```python
from build123d import *

# Parameters (mm, degrees)
PAD_DEPTH         = 6
PAD001_DEPTH      = 2
PAD002_DEPTH      = 100
SKETCH003_W       = 2.4
SKETCH003_H       = 10
POCKET_DEPTH      = 2.351
POCKET_DEPTH_BACK = -2.351
PAD003_DEPTH      = 10


with BuildPart() as part:
    # Sketch → Pad (new body)
    with BuildSketch(Plane.XY):
        with BuildLine():
            ThreePointArc((-2.3, 2.35), (-3.288237, 0), (-2.3, -2.35))
            Line((-2.3, -2.35), (2.3, -2.35))
            ThreePointArc((2.3, -2.35), (3.288237, 0), (2.3, 2.35))
            Line((-2.3, 2.35), (2.3, 2.35))
        make_face()
        with BuildLine():
            ThreePointArc((1.341641, -1.55), (2.05, 0), (1.341641, 1.55))
            Line((-1.341641, 1.55), (1.341641, 1.55))
            ThreePointArc((-1.341641, 1.55), (-2.05, 0), (-1.341641, -1.55))
            Line((1.341641, -1.55), (-1.341641, -1.55))
        make_face(mode=Mode.SUBTRACT)
    extrude(amount=PAD_DEPTH)

    # Sketch001 → Pad001 (join)
    with BuildSketch(Plane.XY):
        with BuildLine():
            ThreePointArc((-2.3, 2.3), (-3.252691, 0), (-2.3, -2.3))
            Line((-2.3, -2.3), (2.3, -2.3))
            ThreePointArc((2.3, -2.3), (3.252691, 0), (2.3, 2.3))
            Line((-2.3, 2.3), (2.3, 2.3))
        make_face()
    extrude(amount=-PAD001_DEPTH)

    # Sketch002 → Pad002 (join)
    with BuildSketch(Plane.XY.offset(-2)):
        Polygon((-0.8, 2.35), (-0.8, -0.75), (-2.3, -0.75), (-2.3, -2.35), (2.3, -2.35), (2.3, -0.75), (0.8, -0.75), (0.8, 2.35), align=None)
    extrude(amount=-PAD002_DEPTH)

    # Sketch003 → Pocket (cut, two sides)
    with BuildSketch(Plane.XZ) as pocket_sk:
        with Locations((0, 5)):
            Rectangle(SKETCH003_W, SKETCH003_H)
    extrude(amount=-POCKET_DEPTH, mode=Mode.SUBTRACT)
    extrude(pocket_sk.sketch, amount=-POCKET_DEPTH_BACK, mode=Mode.SUBTRACT)

    # Sketch004 → Pad003 (join)
    with BuildSketch(Plane.XY.offset(-102)):
        with BuildLine():
            ThreePointArc((2.12132, 4.12132), (2.771639, 5.09459), (3, 6.242641))
            Line((3, 16.242641), (3, 6.242641))
            ThreePointArc((3, 16.242641), (2.771639, 17.390691), (2.12132, 18.363961))
            Line((2.12132, 18.363961), (1.375736, 19.109545))
            ThreePointArc((2.224264, 19.958074), (1.375736, 19.958074), (1.375736, 19.109545))
            Line((2.969848, 19.212489), (2.224264, 19.958074))
            ThreePointArc((4.2, 16.242641), (3.880294, 17.849911), (2.969848, 19.212489))
            Line((4.2, 16.242641), (4.2, 6.242641))
            ThreePointArc((2.969848, 3.272792), (3.880294, 4.63537), (4.2, 6.242641))
            Line((2.969848, 3.272792), (0, 0.302944))
            Line((0, 2), (0, 0.302944))
            Line((2.12132, 4.12132), (0, 2))
        make_face()
    pad003 = extrude(amount=PAD003_DEPTH)

    # Mirrored: Pad003 across Sketch004 V_Axis
    add(pad003.mirror(Plane(origin=(0, 0, -102), x_dir=(0, 0, 1), z_dir=(1, 0, 0))))


solid = part.part
```
Input: part model. Units: mm. Frame: model coordinates. A direction names the side the tool comes from. Give positions to 0.01 mm unless a question says otherwise; leave off trailing zeros. Order: outer loops, then holes, each group sorted by start corner. A loop starts at its lowest first (then second) coordinate and runs counter-clockwise, first axis right, second up. Notation, with made-up numbers: M -25,-5 L 15,-5 A18 ccw 15,0 Z; hole C 8,8 d8. An arc over 180 degrees is marked long. Return JSON: item names as keys, results as strings.
1) Contact query for flat-ended pins moving along their axis: pin 1 (6 mm diameter, centred on y = 6.5, z = -21, fed in from +X); pin 2 (4.5 mm diameter, centred on x = 0, y = -0.5, fed in from +Z); pin 3 (0.5 mm diameter, centred on y = -1.5, z = -65, fed in from +X); pin 4 (0.9 mm diameter, centred on y = 2, z = 2, fed in from +X). Output: stop coordinate, or through.
Taken from the geometry:
{"pin 1": "passes through", "pin 2": "stops at z = 6", "pin 3": "stops at x = 2.3", "pin 4": "stops at x = 2.9"}
2) Section query C-C on y = 17.25. Output: boundary loops of the cut face in (x, z).
Taken from the geometry:
{"outline": "M -4.08,-102 L -2.83,-102 L -2.83,-92 L -4.08,-92 Z; M 2.83,-102 L 4.08,-102 L 4.08,-92 L 2.83,-92 Z"}
3) Access query for faces 1 (the face through (-1.9, 2.203, -97.07)), 2 (the face through (0, -2.35, -51)), 3 (the face through (3, 11, -97)). Directions: +Z, -Z, +X, -X, +Y, -Y. A direction counts if a zero-diameter tool reaches every point of the face in a straight line with its end or side. Return the directions, or none.
Taken from the geometry:
{"face 1": "-Z, -X", "face 2": "+Z, -Z, +X, -X, -Y", "face 3": "+Z, -Z"}
4) Line query: L1, parallel to X at y = 10.25, z = -95.5; L2, parallel to Y at x = 1.75, z = -94; L3, parallel to Z at x = 3, y = 18.5. Output: solid intervals per line, ascending. Write a range as [from, to].
Taken from the geometry:
{"L1": "x = [-4.2, -3], [3, 4.2]", "L2": "y = [-2.35, -0.75], [2.05, 3.75], [18.74, 20.13]", "L3": "z = [-102, -92]"}
5) Mould query, pull axis X, two halves, no side actions, for faces 4 (the face through (3.252, -0.036, -0.986)), 5 (the face through (-2, 1, -2)), 6 (the face through (2.778, 17.375, -97.07)). Classes: released by +X, released by -X, zero draft, split by the parting line, or undercut.
Taken from the geometry:
{"face 4": "released by +X", "face 5": "zero draft", "face 6": "undercut"}
6) Section query B-B on z = -6. Output: boundary loops of the cut face in (x, y), and give its area (3 significant figures).
Taken from the geometry:
{"outline": "M -2.3,-2.35 L 2.3,-2.35 L 2.3,-0.75 L 0.8,-0.75 L 0.8,2.35 L -0.8,2.35 L -0.8,-0.75 L -2.3,-0.75 Z", "area": "12.3 mm2"}
7) Section query A-A on y = 13. Output: boundary loops of the cut face in (x, z).
Taken from the geometry:
{"outline": "M -4.2,-102 L -3,-102 L -3,-92 L -4.2,-92 Z; M 3,-102 L 4.2,-102 L 4.2,-92 L 3,-92 Z"}
